Model file for the job. Use its own axes, mm. Round coordinates to 2 decimals unless told otherwise and drop trailing zeros. Loops run counter-clockwise (first coordinate to the right, second up) from the corner with the lowest first, then second, coordinate; pieces in that order, holes last. Notation, with made-up numbers: M -24,-11.5 L 34,-11.5 A27 ccw 34,11.5 Z; hole C 3,-29 d9. An arc over 180 degrees is marked long. Use a Markdown table: item, result. Add a question column.
Q1. Probe line 1 (X direction, y = 0.5, z = 1.75); line 2 (Y direction, x = -44, z = 7.7); line 3 (X direction, y = -1.25, z = 1.5). List the from-to ranges inside material, lowest first. Write a range as from..to.
Q2. Pin check, flat tips, straight feed: pin 1 (1.5 mm diameter, centred on y = 3, z = 2, fed in from +X); pin 2 (2 mm diameter, centred on x = -9.5, y = 3, fed in from +Z); pin 3 (4 mm diameter, centred on y = 1, z = 7.5, fed in from +X). Stop position of each tip, or through.
Q3. Cut at B-B (z = 3.25). Give the cut face in (x, y) (3 decimals).
Q4. Cut at A-A (y = 0). Give the cut face in (x, z) (3 decimals).
Q5. Cut at C-C (x = -12.5). Give the cut face in (y, z), plus the area to 3 significant figures.
Q6. Cut at D-D (z = 5.5). Give the cut face in (x, y), plus the area to 3 significant figures.
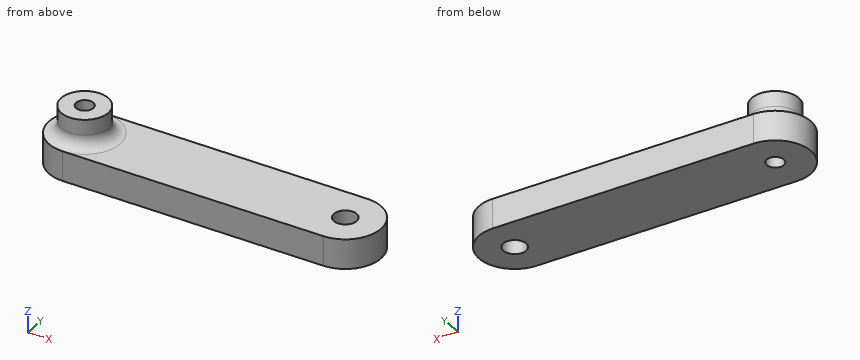
from build123d import *

# Parameters (mm, degrees)
F0_R          = 1.925
F1_DEPTH      = 5
F2_R          = 3.95
F2_R_2        = 1.45
F3_DEPTH      = 4.6
F3_DEPTH_BACK = 5
F4_R          = 2


with BuildPart() as f1:
    # F0 (on Top) → F1 (new body)
    with BuildSketch(Plane.XY):
        with BuildLine():
            Line((-44, -6), (0, -6))
            ThreePointArc((0, -6), (6, 0), (0, 6))
            Line((0, 6), (-44, 6))
            ThreePointArc((-44, 6), (-50, 0), (-44, -6))
        make_face()
        with Locations((-44, 0)):
            Circle(F0_R, mode=Mode.SUBTRACT)
        Circle(F0_R, mode=Mode.SUBTRACT)
    extrude(amount=F1_DEPTH)

    # F2 (on face) → F3 (join, two sides)
    with BuildSketch(Plane.XY.offset(5)) as f3_sk:
        with Locations((-44, 0)):
            Circle(F2_R)
        with Locations((-44, 0)):
            Circle(F2_R_2, mode=Mode.SUBTRACT)
    extrude(amount=F3_DEPTH)
    extrude(f3_sk.sketch, amount=-F3_DEPTH_BACK)

    # F4
    f4_edges = [f1.edges().sort_by_distance(p)[0] for p in [
        (-47.95, 0, 5),
    ]]
    fillet(f4_edges, radius=F4_R)


solid = f1.part
Checked values:
| question | item | result |
|---|---|---|
| 1 | line 1 | x = -49.98..-45.36, -42.64..-1.86, 1.86..5.98 |
| 1 | line 2 | y = -3.95..-1.45, 1.45..3.95 |
| 1 | line 3 | x = -49.87..-44.73, -43.27..-1.46, 1.46..5.87 |
| 2 | pin 1 | stops at x = 5.56 |
| 2 | pin 2 | stops at z = 5 |
| 2 | pin 3 | stops at x = -39.45 |
| 3 | outline | M -44,-6 L 0,-6 A6 ccw 0,6 L -44,6 A6 ccw Z; hole C -44,0 d2.9; hole C 0,0 d3.85 |
| 4 | outline | M -50,0 L -45.45,0 L -45.45,9.6 L -47.95,9.6 L -47.95,7 A2 cw -49.95,5 L -50,5 Z; M -42.55,0 L -1.925,0 L -1.925,5 L -38.05,5 A2 cw -40.05,7 L -40.05,9.6 L -42.55,9.6 Z; M 1.925,0 L 6,0 L 6,5 L 1.925,5 Z |
| 5 | outline | M -6,0 L 6,0 L 6,5 L -6,5 Z |
| 5 | area | 60.0 mm^2 |
| 6 | outline | C -44,0 d9.25; hole C -44,0 d2.9 |
| 6 | area | 60.7 mm^2 |
